Verification items for the finished model (mm, model axes). Round coordinates to 2 decimals unless told otherwise and drop trailing zeros. Write each loop counter-clockwise with the first axis right and the second up, starting at its lowest first coordinate (ties: lowest second). Pieces come first, ordered by that corner, then holes. Notation, with made-up numbers: M 60.5,7.5 L 102.5,7.5 A21 ccw 102.5,14.5 Z; hole C 61,-15 d3. An arc over 180 degrees is marked long. Use a Markdown table: item, result. Add a question column.
from build123d import *

# Parameters (mm, degrees)
SKETCH1_R           = 1.65
BOSS_EXTRUDE1_DEPTH = 1


with BuildPart() as part:
    # Sketch1 → Boss-Extrude1 (new body)
    with BuildSketch(Plane(origin=(0, 0, 0), x_dir=(1, 0, 0), z_dir=(0, 1, 0))):
        with BuildLine():
            Line((0, 2), (0, 33))
            ThreePointArc((0, 33), (0.585786438, 34.414213562), (2, 35))
            Line((2, 35), (9.778174593, 35))
            ThreePointArc((9.778174593, 35), (10.543541458, 34.847759065), (11.192388155, 34.414213562))
            Line((11.192388155, 34.414213562), (34.414213562, 11.192388155))
            ThreePointArc((34.414213562, 11.192388155), (34.847759065, 10.543541458), (35, 9.778174593))
            Line((35, 9.778174593), (35, 2))
            ThreePointArc((35, 2), (34.414213562, 0.585786438), (33, 0))
            Line((33, 0), (2, 0))
            ThreePointArc((2, 0), (0.585786438, 0.585786438), (0, 2))
        make_face()
        with Locations(Location((7.5, 7.5, 0), (0, 0, 270))):
            Circle(SKETCH1_R, mode=Mode.SUBTRACT)
        with Locations(Location((7.5, 27.5, 0), (0, 0, 270))):
            Circle(SKETCH1_R, mode=Mode.SUBTRACT)
        with Locations(Location((17.5, 7.5, 0), (0, 0, 270))):
            Circle(SKETCH1_R, mode=Mode.SUBTRACT)
        with Locations(Location((27.5, 7.5, 0), (0, 0, 270))):
            Circle(SKETCH1_R, mode=Mode.SUBTRACT)
        with Locations(Location((7.5, 17.5, 0), (0, 0, 270))):
            Circle(SKETCH1_R, mode=Mode.SUBTRACT)
        with Locations(Location((17.5, 17.5, 0), (0, 0, 270))):
            Circle(SKETCH1_R, mode=Mode.SUBTRACT)
    extrude(amount=BOSS_EXTRUDE1_DEPTH)


solid = part.part
1. Scan lines: line 1 along X through (y, z) = (0.4, -7.5); line 2 along X through (y, z) = (0.9, -6); line 3 along Z through (x, y) = (6, 0.1). Record each from-to range of solid material in increasing order. Write a range as from..to.
2. Cross-section at D-D on z = -27.5. Enter the section's corners in (x, y).
3. Cross-section at B-B on z = -7.5. Enter the section's corners in (x, y), plus the area to 3 significant figures.
4. Release check for a two-part mould opening along Z. For faces 1 (the cylindrical face through (10.533, 0.493, -34.852)), 2 (the cylindrical face through (6.5, 0.49, -18.81)), 3 (the flat face through (17.7, 0.5, 0)) record: +Z half, -Z half, draft (parallel to the pull), parting line (faces both ways), or undercut.
5. Cross-section at C-C on y = 0.7. Enter the section's corners in (x, z).
6. Cross-section at A-A on x = 7.5. Enter the section's corners in (y, z), plus the area to 3 significant figures.
Answer:
| question | item | result |
|---|---|---|
| 1 | line 1 | x = 0..5.85, 9.15..15.85, 19.15..25.85, 29.15..35 |
| 1 | line 2 | x = 0..6.81, 8.19..16.81, 18.19..26.81, 28.19..35 |
| 1 | line 3 | z = -35..-28.19, -26.81..-18.19, -16.81..-8.19, -6.81..0 |
| 2 | outline | M 0,0 L 5.85,0 L 5.85,1 L 0,1 Z; M 9.15,0 L 18.11,0 L 18.11,1 L 9.15,1 Z |
| 3 | outline | M 0,0 L 5.85,0 L 5.85,1 L 0,1 Z; M 9.15,0 L 15.85,0 L 15.85,1 L 9.15,1 Z; M 19.15,0 L 25.85,0 L 25.85,1 L 19.15,1 Z; M 29.15,0 L 35,0 L 35,1 L 29.15,1 Z |
| 3 | area | 25.1 mm^2 |
| 4 | face 1 | -Z half |
| 4 | face 2 | undercut |
| 4 | face 3 | +Z half |
| 5 | outline | M 0,-33 A2 ccw 2,-35 L 9.78,-35 A2 ccw 11.19,-34.41 L 34.41,-11.19 A2 ccw 35,-9.78 L 35,-2 A2 ccw 33,0 L 2,0 A2 ccw 0,-2 Z; hole C 7.5,-27.5 d3.3; hole C 7.5,-17.5 d3.3; hole C 7.5,-7.5 d3.3; hole C 17.5,-17.5 d3.3; hole C 17.5,-7.5 d3.3; hole C 27.5,-7.5 d3.3 |
| 6 | outline | M 0,-35 L 1,-35 L 1,-29.15 L 0,-29.15 Z; M 0,-25.85 L 1,-25.85 L 1,-19.15 L 0,-19.15 Z; M 0,-15.85 L 1,-15.85 L 1,-9.15 L 0,-9.15 Z; M 0,-5.85 L 1,-5.85 L 1,0 L 0,0 Z |
| 6 | area | 25.1 mm^2 |
